from build123d import *

# Parameters (mm, degrees)
EXTRUDE_1_DEPTH     = 5.5
SKETCH_2_W          = 5.5
SKETCH_2_H          = 7.5
CUT_EXTRUDE_1_DEPTH = 39.432591177


with BuildPart() as part:
    # ｽｹｯﾁ1 → ﾎﾞｽ - 押し出し1 (new body)
    with BuildSketch(Plane.XY):
        with BuildLine():
            Line((-10, 15.682575771), (-10, 0))
            Line((-10, 0), (10, 0))
            Line((10, 0), (10, 15.682575771))
            ThreePointArc((10, 15.682575771), (16.156067067, 19.752281924), (20.784609691, 25.5))
            ThreePointArc((20.784609691, 25.5), (19.320508076, 30.964101615), (13.856406461, 29.5))
            ThreePointArc((13.856406461, 29.5), (0, 21.5), (-13.856406461, 29.5))
            ThreePointArc((-13.856406461, 29.5), (-19.320508076, 30.964101615), (-20.784609691, 25.5))
            ThreePointArc((-20.784609691, 25.5), (-16.156067067, 19.752281924), (-10, 15.682575771))
        make_face()
    extrude(amount=EXTRUDE_1_DEPTH)

    # ｽｹｯﾁ2 → ｶｯﾄ - 押し出し1 (cut, through all)
    with BuildSketch(Plane.XY.offset(5.5)):
        with Locations((7.25, 3.75)):
            Rectangle(SKETCH_2_W, SKETCH_2_H)
        with Locations((-7.25, 3.75)):
            Rectangle(SKETCH_2_W, SKETCH_2_H)
    extrude(amount=-CUT_EXTRUDE_1_DEPTH, mode=Mode.SUBTRACT)


solid = part.part
Here's how the part is built. I have some questions about the finished solid (model axes, mm). A direction names the side the tool comes from. Round coordinates to 2 decimals unless told otherwise and drop trailing zeros. Loops run counter-clockwise (first coordinate to the right, second up) from the corner with the lowest first, then second, coordinate; pieces in that order, holes last.
1. We'd pull the mould along X, two halves only. Please class faces 1 (the face through (0.2, 21.5, 2.7)), 2 (the face through (-7, 7.5, 3)), 3 (the face through (-16.23, 19.82, 2.71)): +X half, -X half, draft (parallel to the pull), parting line (faces both ways), or undercut.
Answer list:
face 1: undercut
face 2: draft
face 3: -X half
2. Which directions (+Z, -Z, +X, -X, +Y, -Y) give clear straight access to the entire face, cutting with the end or side of a thin tool? Please do faces 4 (the face through (-4.5, 4, 3)), 5 (the face through (4.5, 4, 3)), 6 (the face through (0, 0, 3)).
Answer list:
face 4: +Z, -Z, -X, -Y
face 5: +Z, -Z, +X, -Y
face 6: +Z, -Z, +X, -X, -Y
3. If we section it at D-D on x = 1: Write out the boundary of the cut face in (y, z), plus the area to 3 significant figures.
Answer list:
outline: (0, 0) - (21.53, 0) - (21.53, 5.5) - (0, 5.5) - close
area: 118 mm2
4. For P1, Ø1, axis at x = 5, z = 1.5, coming from the +Y side (3 decimals); P2, Ø1.6, axis at y = 11, z = 3, coming from the +X side; P3, Ø1.5, axis at x = -17, z = 4.5, coming from the -Y side; P4, Ø10, axis at x = 3, y = 28, coming from the +Z side, each with a flat end and sliding along its axis, tell me the tip position at first contact or that it passes through.
Answer list:
P1: stops at y = 22.475
P2: stops at x = 10
P3: stops at y = 19.84
P4: passes through
5. If we section it at B-B on z = 1.95: Write out the boundary of the cut face in (x, y).
Answer list:
outline: (-20.78, 25.5) arc R24 ccw to (-10, 15.68) - (-10, 7.5) - (-4.5, 7.5) - (-4.5, 0) - (4.5, 0) - (4.5, 7.5) - (10, 7.5) - (10, 15.68) arc R24 ccw to (20.78, 25.5) arc R4 ccw to (13.86, 29.5) arc R16 cw to (-13.86, 29.5) arc R4 ccw to start
6. If we section it at C-C on y = 6: Write out the boundary of the cut face in (x, z).
Answer list:
outline: (-4.5, 0) - (4.5, 0) - (4.5, 5.5) - (-4.5, 5.5) - close
7. If we section it at A-A on y = 27.5: Write out the boundary of the cut face in (x, z).
Answer list:
outline: (-21.32, 0) - (-12.49, 0) - (-12.49, 5.5) - (-21.32, 5.5) - close; (12.49, 0) - (21.32, 0) - (21.32, 5.5) - (12.49, 5.5) - close
8. If I drill on line 1 along X through (y, z) = (8.5, 1.4); line 2 along X through (y, z) = (24, 1.8); line 3 along X through (y, z) = (30, 1.7), over which ranges is the centre line in solid material (lowest first)?
Answer list:
line 1: x = -10 to 10
line 2: x = -19.84 to -8.59, 8.59 to 19.84
line 3: x = -20.44 to -14.2, 14.2 to 20.44
